```python
from build123d import *

# Parameters (mm, degrees)
ESBO_O1_W                  = 300
ESBO_O1_H                  = 400
ESBO_O1_R                  = 13
EXTRUS_O1_DEPTH            = 34
FURO_ROSCADO_DE_M161_D     = 14
FURO_ROSCADO_DE_M161_DEPTH = 28
FURO_ROSCADO_DE_M161_TIP   = 4.206024333
FURO1_D                    = 42
FURO1_CBORE_D              = 48
FURO1_CBORE_DEPTH          = 8


with BuildPart() as part:
    # Esboço1 → Extrusão1 (new body)
    with BuildSketch(Plane(origin=(0, 0, 0), x_dir=(1, 0, 0), z_dir=(0, 1, 0))):
        Rectangle(ESBO_O1_W, ESBO_O1_H)
        with Locations(Location((0, 0, 0), (0, 0, 270))):  # turned: the seam where the file's is
            Circle(ESBO_O1_R, mode=Mode.SUBTRACT)
    extrude(amount=EXTRUS_O1_DEPTH)

    # Furo roscado de M161
    with Locations(Plane.XZ):
        with Locations((-118, 119), (118, 119), (-118, -119), (118, -119)):
            Hole(FURO_ROSCADO_DE_M161_D / 2, depth=FURO_ROSCADO_DE_M161_DEPTH)
            with Locations((0, 0, -(FURO_ROSCADO_DE_M161_DEPTH + FURO_ROSCADO_DE_M161_TIP / 2))):  # 118° drill point
                Cone(0, FURO_ROSCADO_DE_M161_D / 2, FURO_ROSCADO_DE_M161_TIP, mode=Mode.SUBTRACT)

    # Furo1 (through all)
    with Locations(Plane.XZ):
        with Locations((118, 168), (118, -168), (-118, -168), (-118, 168)):
            CounterBoreHole(FURO1_D / 2, FURO1_CBORE_D / 2, FURO1_CBORE_DEPTH)


solid = part.part
```
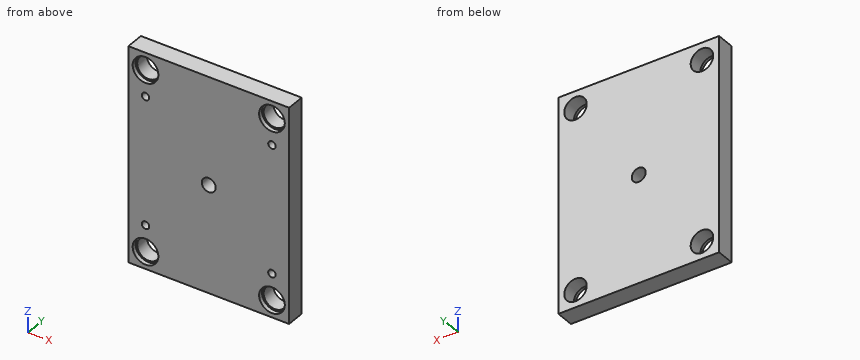
The listing builds one solid part. Answer for the finished solid, in the listing's coordinates (mm). Give positions to 0.01 mm unless a question says otherwise; leave off trailing zeros. Order: outer loops, then holes, each group sorted by start corner. A loop starts at its lowest first (then second) coordinate and runs counter-clockwise, first axis right, second up. Notation, with made-up numbers: (-24, -32) - (2, -32) arc R10 ccw to (2, -13) - close; hole circle Ø10 at (-19, -16.75). An arc over 180 degrees is marked (long way). Use one line per item in the form item = value. Start each with the question number.
(1) A cutting plane is placed at B-B, the plane z = 168. Write down the section's boundary in (x, y), then the cut area to 3 significant figures.
(2) A cutting plane is placed at A-A, the plane x = 0. Write down the section's boundary in (y, z), then the cut area to 3 significant figures.
(3) Flat-ended cylindrical pins translate along their axes: pin 1 Ø8.5 at (x, z) = (-118, 119) entering from -Y; pin 2 Ø12.5 at (x, z) = (-118, -119) entering from -Y; pin 3 Ø8 at (x, z) = (-118, 120.5) entering from -Y. Find the tip coordinate at first contact, or state that the pin passes through.
(4) Consider line 1 (Z direction, x = 118, y = 21); line 2 (Z direction, x = -118, y = 2); line 3 (Z direction, x = 107, y = 22). Determine where each line is inside the solid, lowest interval first. Write a range as from..to.
Ans:
q1.outline = (-150, 0) - (-142, 0) - (-142, 8) - (-139, 8) - (-139, 34) - (-150, 34) - close; (-97, 8) - (-94, 8) - (-94, 0) - (94, 0) - (94, 8) - (97, 8) - (97, 34) - (-97, 34) - close; (139, 8) - (142, 8) - (142, 0) - (150, 0) - (150, 34) - (139, 34) - close
q1.area = 7,250 mm^2
q2.outline = (0, -200) - (34, -200) - (34, -13) - (0, -13) - close; (0, 13) - (34, 13) - (34, 200) - (0, 200) - close
q2.area = 12,700 mm^2
q3.pin_1 = 29.65
q3.pin_2 = 28.45
q3.pin_3 = 28.9
q4.line_1 = -200..-189, -147..-126, -112..112, 126..147, 189..200
q4.line_2 = -200..-192, -144..-126, -112..112, 126..144, 192..200
q4.line_3 = -200..-185.89, -150.11..150.11, 185.89..200
